The model under review builds one solid part; all positions refer to its coordinate system, in mm. A direction names the side the tool comes from. Round coordinates to 2 decimals unless told otherwise and drop trailing zeros. Order: outer loops, then holes, each group sorted by start corner. A loop starts at its lowest first (then second) coordinate and runs counter-clockwise, first axis right, second up. Notation, with made-up numbers: (-25, -27) - (-5, -27) arc R24 cw to (-5, 4) - close; hole circle Ø8 at (45, -35.5). An arc over 180 degrees is marked (long way). One line per question, with ' | ' between items. Start each with the question number.
Item 1: Add section A-A on y = -0.75. State the section outline as (x, z) points.
Item 2: Tool access review of faces 4 (the face through (-6, -3, 5)), 5 (the face through (-6.63, -1.48, 3.29)): name each direction out of +Z, -Z, +X, -X, +Y, -Y from which nothing blocks a thin tool from reaching the whole face with its end or side.
Item 3: Add section B-B on x = 6.25. State the section outline as (y, z) points.
Item 4: Draft analysis for pull direction X (two halves, no side actions). For faces 1 (the face through (12.5, 1, -10)), 2 (the face through (0, 1, 10)), 3 (the face through (5.87, -1.48, 3.29)), state which applies: +X half, -X half, draft (parallel to the pull), parting line (faces both ways), or undercut.
Item 5: Add section D-D on z = -2.5. State the section outline as (x, y) points.
Item 6: Insertion check: pin 1 Ø2 at (x, y) = (-0.5, -2) entering from -Z; pin 2 Ø1.5 at (x, y) = (8.5, -1.5) entering from +Z. Each pin has a flat end and moves straight along its axis. Give the tip position at first contact, or say it passes through.
Item 7: For L1, parallel to Y at x = -9.75, z = -17; L2, parallel to X at y = -0.45, z = 6; L3, parallel to Z at x = 5, y = -2.5, list the stretches that pass through material, from the lowest coordinate up. Write a range as [from, to].
Item 8: Add section C-C on z = 5. State the section outline as (x, y) points.
from build123d import *

# Parameters (mm, degrees)
F0_W     = 25
F0_H     = 40
F0_R     = 1.75
F1_DEPTH = 3
F2_DEPTH = 3


with BuildPart() as f1:
    # F0 (on Front) → F1 (new body)
    with BuildSketch(Plane.XZ):
        with Locations((0, -10)):
            Rectangle(F0_W, F0_H)
        with Locations((-6.25, 5)):
            Circle(F0_R, mode=Mode.SUBTRACT)
        with Locations((6.25, 5)):
            Circle(F0_R, mode=Mode.SUBTRACT)
        with Locations((-6.25, 5)):
            Circle(F0_R)
        with Locations((6.25, 5)):
            Circle(F0_R)
    extrude(amount=-F1_DEPTH)

    # F0 (on Front) → F2 (join)
    with BuildSketch(Plane.XZ):
        with Locations((-6.25, 5)):
            Circle(F0_R)
        with Locations((6.25, 5)):
            Circle(F0_R)
    extrude(amount=F2_DEPTH)


solid = f1.part
Determined:
1) outline: circle Ø3.5 at (-6.25, 5); circle Ø3.5 at (6.25, 5)
2) face 4: +Z, -Z, +X, -X, -Y | face 5: -Y
3) outline: (-3, 3.25) - (0, 3.25) - (0, -30) - (3, -30) - (3, 10) - (0, 10) - (0, 6.75) - (-3, 6.75) - close
4) face 1: +X half | face 2: draft | face 3: undercut
5) outline: (-12.5, 0) - (12.5, 0) - (12.5, 3) - (-12.5, 3) - close
6) pin 1: through | pin 2: z = 5.9
7) L1: [0, 3] | L2: [-7.69, -4.81], [4.81, 7.69] | L3: [3.78, 6.22]
8) outline: (-12.5, 0) - (-8, 0) - (-8, -3) - (-4.5, -3) - (-4.5, 0) - (4.5, 0) - (4.5, -3) - (8, -3) - (8, 0) - (12.5, 0) - (12.5, 3) - (-12.5, 3) - close
